Input: dimensioned drawing with shaded views. Units: mm. Origin: part minimum x, y, z. A direction names the side the tool comes from. Round coordinates to 2 decimals unless told otherwise and drop trailing zeros. Loops run counter-clockwise (first coordinate to the right, second up) from the corner with the lowest first, then second, coordinate; pieces in that order, holes last. Notation, with made-up numbers: (-2.5, 37) - (51.5, 37) arc R35 cw to (51.5, 76) - close; hole circle Ø11 at (70.5, 64). An arc over 180 degrees is marked (long way). Answer as a JSON object with one key per item and string values. Group by question number.
Item 1: Section B-B (y = 2). Return the cut outline in (x, z), plus the area to 3 significant figures.
Item 2: Section D-D (y = 3.75). Return the cut outline in (x, z) (3 decimals).
Item 3: Section A-A (z = 6). Return the cut outline in (x, y) (3 decimals), plus the area to 3 significant figures.
Item 4: Reachability of the marked faces 1 and 2 from +Z, -Z, +X, -X, +Y, -Y: full face, straight path, thin tool, end or side. Return the list, or none.
Item 5: Section C-C (x = 10.25). Return the cut outline in (y, z).
Item 6: Line query: line 1 (Y direction, x = 3, z = 2); line 2 (X direction, y = 6, z = 4); line 3 (Z direction, x = 5.25, y = 3.5). Output: solid intervals per line, ascending.
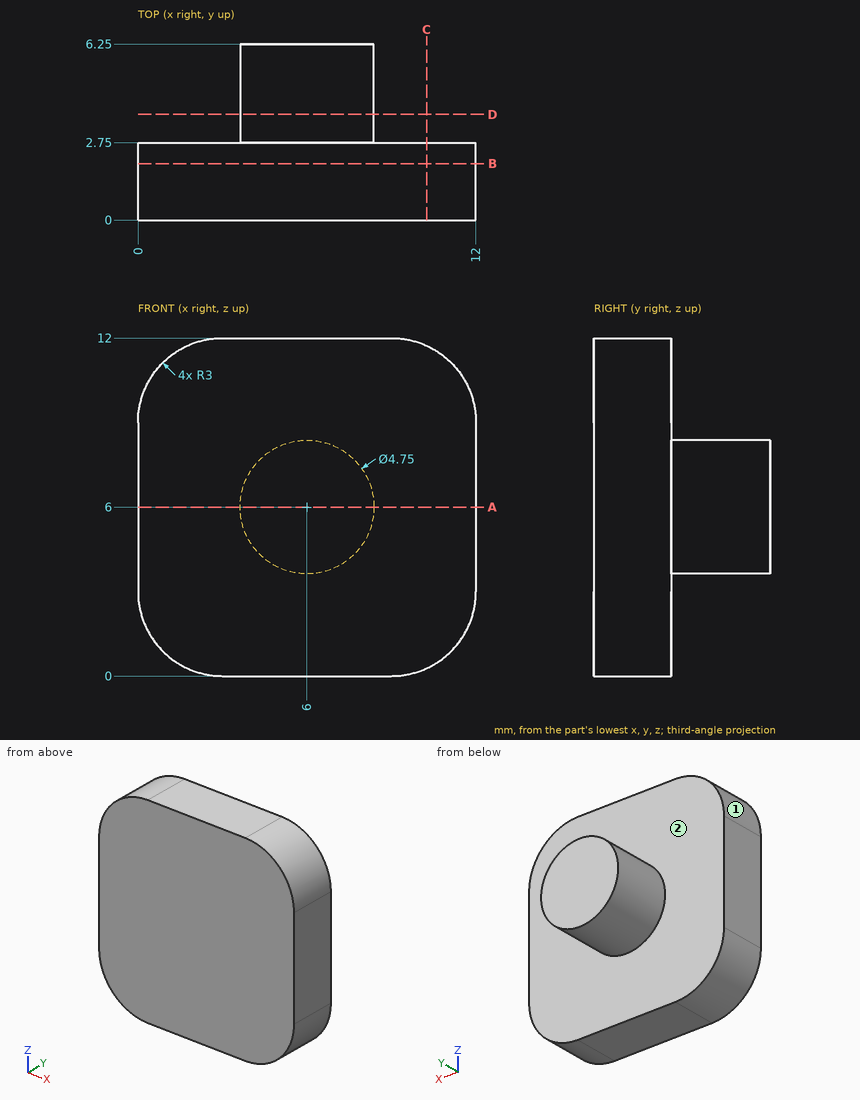
Values:
{
 "1": {"outline": "(0, 3) arc R3 ccw to (3, 0) - (9, 0) arc R3 ccw to (12, 3) - (12, 9) arc R3 ccw to (9, 12) - (3, 12) arc R3 ccw to (0, 9) - close", "area": "136 mm^2"},
 "2": {"outline": "circle Ø4.75 at (6, 6)"},
 "3": {"outline": "(0, 0) - (12, 0) - (12, 2.75) - (8.375, 2.75) - (8.375, 6.25) - (3.625, 6.25) - (3.625, 2.75) - (0, 2.75) - close", "area": "49.6 mm^2"},
 "4": {"face 1": "+Z, -X, +Y, -Y", "face 2": "+Y"},
 "5": {"outline": "(0, 0.27) - (2.75, 0.27) - (2.75, 11.73) - (0, 11.73) - close"},
 "6": {"line 1": "y = 0 to 2.75", "line 2": "x = 4.72 to 7.28", "line 3": "z = 3.75 to 8.25"}
}
